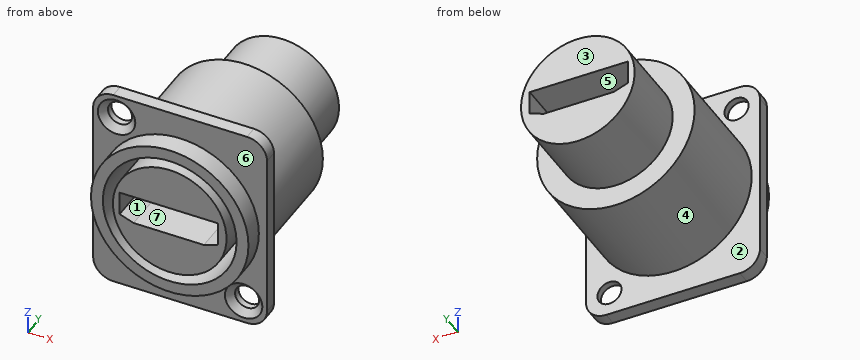
```python
from build123d import *

# Parameters (mm, degrees)
SKETCH1_W           = 26
SKETCH1_H           = 31
EXTRUDE1_DEPTH      = 2
SKETCH2_R           = 11.775
EXTRUDE2_DEPTH      = 3
EXTRUDE2_DEPTH_BACK = 18.5
SKETCH3_R           = 8.5
EXTRUDE3_DEPTH      = 11
SKETCH4_R           = 10
SKETCH4_R_2         = 8.5
EXTRUDE4_DEPTH      = 15
EXTRUDE5_DEPTH      = 10
SKETCH9_R           = 1.8
EXTRUDE6_DEPTH      = 10
CHAMFER1_SIZE       = 1
FILLET1_R           = 3
EXTRUDE7_DEPTH      = 10


with BuildPart() as part:
    # Sketch1 → Extrude1 (new body)
    with BuildSketch(Plane(origin=(0, 0, 0), x_dir=(1, 0, 0), z_dir=(0, 1, 0))):
        with Locations((13, -15.5)):
            Rectangle(SKETCH1_W, SKETCH1_H)
    extrude(amount=EXTRUDE1_DEPTH)

    # Sketch2 → Extrude2 (add, two sides)
    with BuildSketch(Plane(origin=(0, 0, 0), x_dir=(-1, 0, 0), z_dir=(0, -1, 0))) as extrude2_sk:
        with Locations((-13, -15.5)):
            Circle(SKETCH2_R)
    extrude(amount=EXTRUDE2_DEPTH)
    extrude(extrude2_sk.sketch, amount=-EXTRUDE2_DEPTH_BACK)

    # Sketch3 → Extrude3 (add)
    with BuildSketch(Plane(origin=(0, 18.5, 0), x_dir=(1, 0, 0), z_dir=(0, 1, 0))):
        with Locations((13, -15.5)):
            Circle(SKETCH3_R)
    extrude(amount=EXTRUDE3_DEPTH)

    # Sketch4 → Extrude4 (cut)
    with BuildSketch(Plane(origin=(0, -3, 0), x_dir=(-1, 0, 0), z_dir=(0, -1, 0))):
        with Locations((-13, -15.5)):
            Circle(SKETCH4_R)
        with Locations((-13, -15.5)):
            Circle(SKETCH4_R_2, mode=Mode.SUBTRACT)
    extrude(amount=-EXTRUDE4_DEPTH, mode=Mode.SUBTRACT)

    # Sketch5 → Extrude5 (cut)
    with BuildSketch(Plane(origin=(0, -3, 0), x_dir=(-1, 0, 0), z_dir=(0, -1, 0))):
        Polygon((-5.519295113, -14.065487649), (-7.596667184, -13.309386049), (-18.109711193, -13.309386049), (-20.187083264, -14.065487649), (-20.187083264, -17.643859967), (-5.519295113, -17.643859967), align=None)
    extrude(amount=-EXTRUDE5_DEPTH, mode=Mode.SUBTRACT)

    # Sketch9 → Extrude6 (cut)
    with BuildSketch(Plane.XZ):
        with Locations((3.5, 27.5)):
            Circle(SKETCH9_R)
        with Locations((22.5, 3.5)):
            Circle(SKETCH9_R)
    extrude(amount=-EXTRUDE6_DEPTH, mode=Mode.SUBTRACT)

    # Chamfer1
    chamfer1_edges = [part.edges().sort_by_distance(p)[0] for p in [
        (1.7, 0, 27.5),
        (20.7, 0, 3.5),
    ]]
    chamfer(chamfer1_edges, length=CHAMFER1_SIZE)

    # Fillet1
    fillet1_edges = [part.edges().sort_by_distance(p)[0] for p in [
        (0, 1, 0),
        (26, 1, 0),
        (26, 1, 31),
        (0, 1, 31),
    ]]
    fillet(fillet1_edges, radius=FILLET1_R)

    # Sketch10 → Extrude7 (cut)
    with BuildSketch(Plane(origin=(0, 29.5, 0), x_dir=(1, 0, 0), z_dir=(0, 1, 0))):
        Polygon((5.519295113, -14.065487649), (5.519295113, -17.643859967), (20.187083264, -17.643859967), (20.187083264, -14.065487649), (18.109711193, -13.309386049), (7.596667184, -13.309386049), align=None)
    extrude(amount=-EXTRUDE7_DEPTH, mode=Mode.SUBTRACT)


solid = part.part
```
Geometry check sheet. Reference: the model listing, model coordinates, mm. Face numbers are marked on the shaded views. A direction names the side the tool comes from. Coordinates: 2 decimals unless noted, no trailing zeros. Write each loop counter-clockwise with the first axis right and the second up, starting at its lowest first coordinate (ties: lowest second). Pieces come first, ordered by that corner, then holes. Notation, with made-up numbers: M 60,29.25 L 105,29.25 A31 cw 105,55.25 Z; hole C 28.25,41 d11. An arc over 180 degrees is marked long. Answer as a JSON object with one key per item and string values.
1. Section check A-A, the plane y = 4.5. Enter the section's corners in (x, z) (3 decimals).
Answers below:
{"outline": "C 13,15.5 d23.55; C 13,15.5 d17; hole C 13,15.5 d20; hole M 5.519,14.065 L 7.597,13.309 L 18.11,13.309 L 20.187,14.065 L 20.187,17.644 L 5.519,17.644 Z"}
2. Go/stop test with flat-tipped pins: pin 1 Ø3 at (x, z) = (22.5, 3.5) entering from +Y; pin 2 Ø2 at (y, z) = (25.5, 22) entering from +X; pin 3 Ø10 at (x, y) = (21.5, 8) entering from +Z; pin 4 Ø6 at (y, z) = (19, 20) entering from +X. Record where each tip stops, or that it passes through.
Answers below:
{"pin 1": "passes through", "pin 2": "stops at x = 19.48", "pin 3": "stops at z = 26.74", "pin 4": "stops at x = 24.67"}
3. Section check C-C, the plane x = 22.5. Enter the section's corners in (y, z).
Answers below:
{"outline": "M -3,8.54 L 0,8.54 L 0,6.3 L 1,5.3 L 2,5.3 L 2,8.54 L 18.5,8.54 L 18.5,22.46 L 2,22.46 L 2,31 L 0,31 L 0,22.46 L -3,22.46 L -3,18.62 L 12,18.62 L 12,12.38 L -3,12.38 Z; M 0,0 L 2,0 L 2,1.7 L 1,1.7 L 0,0.7 Z"}
4. Scan lines: L1, parallel to Z at x = 13, y = 2.75 (3 decimals); L2, parallel to X at y = 0.25, z = 15.5; L3, parallel to Z at x = 13, y = 1.25. Record each from-to range of solid material in increasing order.
Answers below:
{"L1": "z = 3.725 to 5.5, 7 to 13.309, 17.644 to 24, 25.5 to 27.275", "L2": "x = 0 to 3, 4.5 to 5.52, 20.19 to 21.5, 23 to 26", "L3": "z = 0 to 5.5, 7 to 13.31, 17.64 to 24, 25.5 to 31"}
5. Draft check along X on the marked faces 4, 5, 6 and 7. Enter one of: released by +X, released by -X, zero draft, split by the parting line, or undercut.
Answers below:
{"face 4": "split by the parting line", "face 5": "undercut", "face 6": "zero draft", "face 7": "undercut"}
6. Tool access check on the marked faces 1, 2 and 3. Record the directions out of +Z, -Z, +X, -X, +Y, -Y that give a thin tool (end or side, any length) a straight path to the whole face; none if there is none.
Answers below:
{"face 1": "-Y", "face 2": "+Y", "face 3": "+Z, -Z, +X, -X, +Y"}
